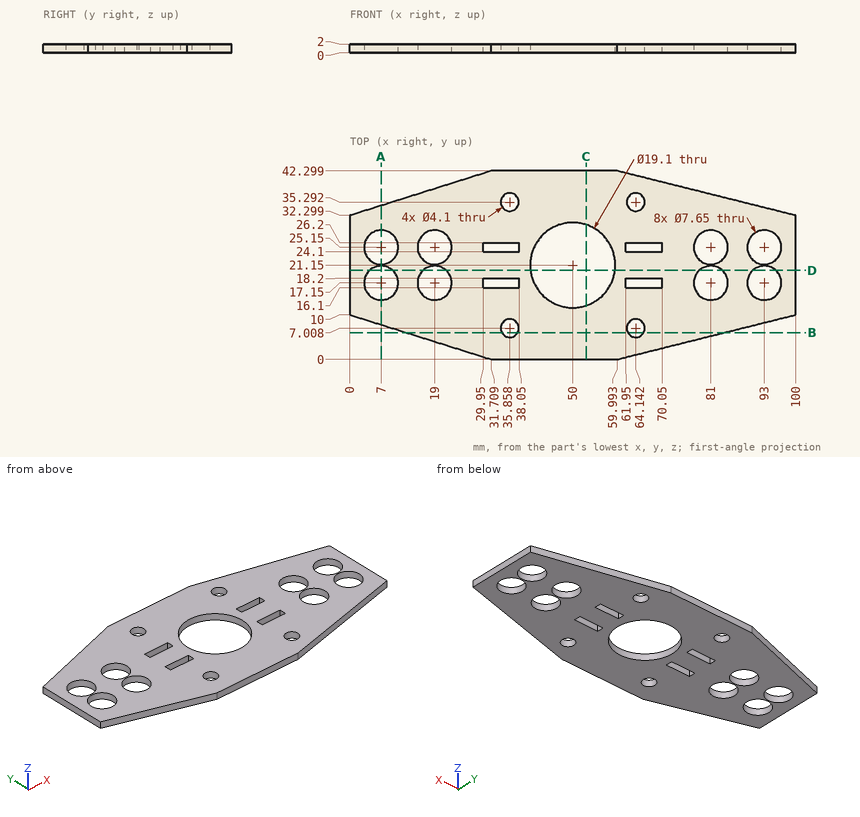
Study the drawing (mm; zero at the part's minimum x, y, z) and answer. Coordinates: 2 decimals unless noted, no trailing zeros. Loops run counter-clockwise (first coordinate to the right, second up) from the corner with the lowest first, then second, coordinate; pieces in that order, holes last. Notation, with made-up numbers: M 78.25,70.5 L 120.25,70.5 A32 cw 120.25,97.5 Z; hole C 62,24 d5. An arc over 180 degrees is marked long. Answer in a Markdown table with one row per item. Add a question column.
1. Consider L1, parallel to Y at x = 7, z = 0.9 (1 decimal); L2, parallel to Y at x = 91.5, z = 0.35 (1 decimal); L3, parallel to X at y = 18.5, z = 0.4 (1 decimal). Determine where each line is inside the solid, lowest interval first.
2. Find section A-A, the plane x = 7. State how many separate pieces and enclosed holes the cut face has.
3. Find section C-C, the plane x = 53. Write down the section's boundary in (y, z).
4. Find section D-D, the plane y = 20. Write down the section's boundary in (x, z), then the cut area to 3 significant figures.
5. Flat-ended cylindrical pins translate along their axes: P1, Ø6, axis at x = 93, y = 25.15, coming from the +Z side; P2, Ø1, axis at x = 66, z = 1.5, coming from the +Y side; P3, Ø0.6, axis at x = 67, z = 0.5, coming from the +Y side; P4, Ø1, axis at x = 64.5, z = 1, coming from the -Y side. Find the tip coordinate at first contact, or state that the pin passes through.
6. Find section B-B, the plane y = 6. Write down the section's boundary in (x, z), then the cut area to 3 significant figures.
Reported:
| question | item | result |
|---|---|---|
| 1 | L1 | y = 7.8 to 13.3, 21 to 21.3, 29 to 34.5 |
| 1 | L2 | y = 7.9 to 13.6, 20.7 to 21.6, 28.7 to 34.4 |
| 1 | L3 | x = 0 to 3.4, 10.6 to 15.4, 22.6 to 40.8, 59.2 to 77.4, 84.6 to 89.4, 96.6 to 100 |
| 2 | separate pieces | 3 |
| 2 | enclosed holes | 0 |
| 3 | outline | M 0,0 L 12.08,0 L 12.08,2 L 0,2 Z; M 30.22,0 L 42.3,0 L 42.3,2 L 30.22,2 Z |
| 4 | outline | M 0,0 L 4.45,0 L 4.45,2 L 0,2 Z; M 9.55,0 L 16.45,0 L 16.45,2 L 9.55,2 Z; M 21.55,0 L 40.52,0 L 40.52,2 L 21.55,2 Z; M 59.48,0 L 78.45,0 L 78.45,2 L 59.48,2 Z; M 83.55,0 L 90.45,0 L 90.45,2 L 83.55,2 Z; M 95.55,0 L 100,0 L 100,2 L 95.55,2 Z |
| 4 | area | 121 mm^2 |
| 5 | P1 | passes through |
| 5 | P2 | stops at y = 40.92 |
| 5 | P3 | stops at y = 40.62 |
| 5 | P4 | stops at y = 1 |
| 6 | outline | M 12.68,0 L 34.07,0 L 34.07,2 L 12.68,2 Z; M 37.64,0 L 62.36,0 L 62.36,2 L 37.64,2 Z; M 65.93,0 L 84,0 L 84,2 L 65.93,2 Z |
| 6 | area | 128 mm^2 |
